Build history of the part. All positions in model axes, mm. A direction names the side the tool comes from. Round coordinates to 2 decimals unless told otherwise and drop trailing zeros. Order: outer loops, then holes, each group sorted by start corner. A loop starts at its lowest first (then second) coordinate and runs counter-clockwise, first axis right, second up. Notation, with made-up numbers: (38.5, 0.25) - (72.5, 0.25) arc R24 cw to (72.5, 37.25) - close; hole circle Ø1 at (89.5, -5). An arc over 180 degrees is marked (long way). One line per question, with ' | ' between items. Start each with the question number.
from build123d import *

# Parameters (mm, degrees)
SKETCH_1_W                   = 86
SKETCH_1_H                   = 80
EXTRUDE_1_DEPTH              = 14
SKETCH_2_R                   = 6
CUT_EXTRUDE_1_DEPTH          = 119.287784661
CUT_EXTRUDE_2_DEPTH          = 2.5
FILLET_1_R                   = 5
HOLE_WIZARD_M6_1_D           = 6.6
HOLE_WIZARD_M6_1_CBORE_D     = 11
HOLE_WIZARD_M6_1_CBORE_DEPTH = 6
HOLE_WIZARD_M5_1_D           = 4.2


with BuildPart() as part:
    # 草图1 → 凸台-拉伸1 (new body)
    with BuildSketch(Plane.XY):
        with Locations((43, 40)):
            Rectangle(SKETCH_1_W, SKETCH_1_H)
    extrude(amount=EXTRUDE_1_DEPTH)

    # 草图2 → 切除-拉伸1 (cut, through all)
    with BuildSketch(Plane.XY.offset(14)):
        with Locations((43, 49)):
            Circle(SKETCH_2_R)
    extrude(amount=-CUT_EXTRUDE_1_DEPTH, mode=Mode.SUBTRACT)

    # 草图3 → 切除-拉伸2 (cut)
    with BuildSketch(Plane.XY.offset(14)):
        Polygon((57, 69), (29, 69), (29, 63), (23, 63), (23, 35), (29, 35), (29, 29), (57, 29), (57, 35), (63, 35), (63, 63), (57, 63), align=None)
    extrude(amount=-CUT_EXTRUDE_2_DEPTH, mode=Mode.SUBTRACT)

    # 圆角1
    fillet_1_edges = [part.edges().sort_by_distance(p)[0] for p in [
        (29, 69, 12.75),
        (57, 69, 12.75),
        (63, 63, 12.75),
        (63, 35, 12.75),
        (57, 29, 12.75),
        (29, 29, 12.75),
        (23, 35, 12.75),
        (23, 63, 12.75),
    ]]
    fillet(fillet_1_edges, radius=FILLET_1_R)

    # M6 六角凹头螺钉的柱形沉头孔1 (through all)
    with Locations(Plane(origin=(0, 80, 0), x_dir=(-1, 0, 0), z_dir=(0, 1, 0))):
        with Locations((-9, 7), (-77, 7)):
            CounterBoreHole(HOLE_WIZARD_M6_1_D / 2, HOLE_WIZARD_M6_1_CBORE_D / 2, HOLE_WIZARD_M6_1_CBORE_DEPTH)

    # M5 螺纹孔1 (through all)
    with Locations(Plane.XY.offset(14)):
        with Locations((68, 74), (18, 74), (18, 24), (68, 24)):
            Hole(HOLE_WIZARD_M5_1_D / 2)


solid = part.part
Item 1: Slice it at A-A (y = 24). Write the cut outline in (x, z).
Item 2: Wall check: line 1 along Y through (x, z) = (68, 4.5); line 2 along Y through (x, z) = (42.5, 6.5); line 3 along Z through (x, y) = (9, 75.5). Give the ranges that are in metal, low to high. Write a range as [from, to].
Item 3: Pull direction Z, two halves, no side cores. Call faces 4 (the face through (5.7, 36.5, 7.1)), 5 (the face through (42, 23, 14)), 6 (the face through (61, 36, 13)), 7 (the face through (73.7, 36.5, 7.1)): released by +Z, released by -Z, zero draft, split by the parting line, or undercut.
Item 4: Slice it at D-D (y = 49). Write the cut outline in (x, z).
Item 5: 3-axis set-ups, long thin cutter, end or side, ignore diameter. For faces 1 (the face through (82.495, 77.042, 7.242)), 2 (the face through (42, 80, 7)), 3 (the face through (31, 68, 13)): which of +Z, -Z, +X, -X, +Y, -Y reach the whole face in a straight line?
Item 6: Slice it at C-C (x = 68). Write the cut outline in (y, z).
Item 7: Slice it at B-B (x = 43). Write the cut outline in (y, z), plus the area to 3 significant figures.
Item 8: Pin check, flat tips, straight feed: pin 1 (10 mm diameter, centred on x = 45, y = 38, fed in from +Z); pin 2 (1 mm diameter, centred on x = 73, z = 6, fed in from +Y). Stop position of each tip, or through.
A:
1) outline: (0, 0) - (15.9, 0) - (15.9, 14) - (0, 14) - close; (20.1, 0) - (65.9, 0) - (65.9, 14) - (20.1, 14) - close; (70.1, 0) - (86, 0) - (86, 14) - (70.1, 14) - close; hole circle Ø6.6 at (9, 7); hole circle Ø6.6 at (77, 7)
2) line 1: [0, 21.9], [26.1, 71.9], [76.1, 80] | line 2: [0, 43.02], [54.98, 80] | line 3: [0, 1.5], [12.5, 14]
3) face 4: undercut | face 5: released by +Z | face 6: zero draft | face 7: undercut
4) outline: (0, 0) - (37, 0) - (37, 11.5) - (23, 11.5) - (23, 14) - (0, 14) - close; (49, 0) - (86, 0) - (86, 14) - (63, 14) - (63, 11.5) - (49, 11.5) - close; hole circle Ø6.6 at (9, 7); hole circle Ø6.6 at (77, 7)
5) face 1: +Y | face 2: +Z, -Z, +X, -X, +Y | face 3: +Z
6) outline: (0, 0) - (21.9, 0) - (21.9, 14) - (0, 14) - close; (26.1, 0) - (71.9, 0) - (71.9, 14) - (26.1, 14) - close; (76.1, 0) - (80, 0) - (80, 14) - (76.1, 14) - close
7) outline: (0, 0) - (43, 0) - (43, 11.5) - (29, 11.5) - (29, 14) - (0, 14) - close; (55, 0) - (80, 0) - (80, 14) - (69, 14) - (69, 11.5) - (55, 11.5) - close | area: 882 mm^2
8) pin 1: z = 11.5 | pin 2: y = 74
